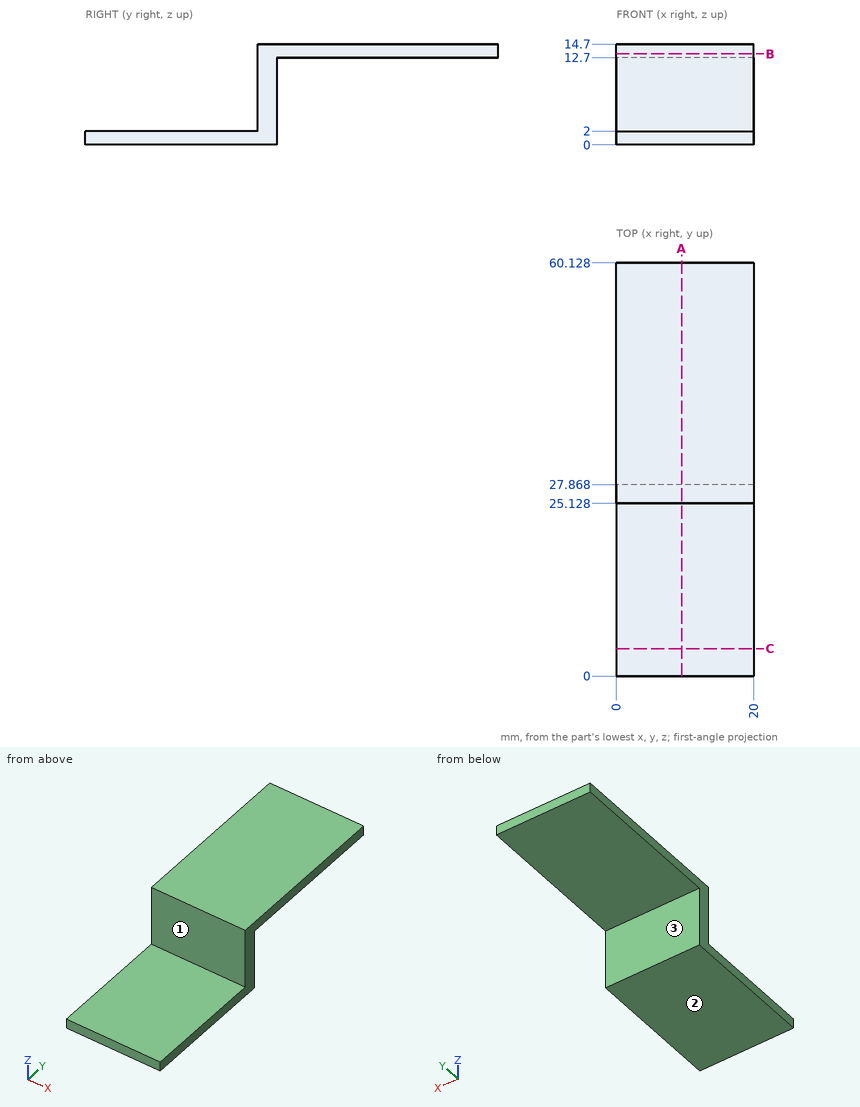
Could you check a few things on this drawing? It's one solid part, dimensions in mm from its lowest x, y, z. A direction names the side the tool comes from. Give positions to 0.01 mm unless a question says otherwise; leave off trailing zeros. Write each loop counter-clockwise with the first axis right and the second up, starting at its lowest first coordinate (ties: lowest second). Pieces come first, ordered by that corner, then holes. Notation, with made-up numbers: M 36,-2.5 L 95,-2.5 A19 cw 95,30.5 Z; hole C -17,57 d1. An arc over 180 degrees is marked long. Put each result on its own line as item: value. Start each with the question number.
Item 1: Will these pins go through, and if not, where does the flat tip stop? pin 1 (10 mm diameter, centred on x = 12, y = 15, fed in from +Z); pin 2 (2 mm diameter, centred on x = 17, z = 4, fed in from -Y); pin 3 (2 mm diameter, centred on x = 3, y = 25, fed in from -Z); pin 4 (6.5 mm diameter, centred on x = 10, z = 7.5, fed in from +Y).
Item 2: On a 3-axis mill with a long thin cutter (end or side, diameter ignored), from which of +Z, -Z, +X, -X, +Y, -Y can I reach the whole of each face in a straight line? I mean the marked faces 1, 2 and 3. Say none if no direction works.
Item 3: If we section it at C-C, the plane y = 4: Write out the boundary of the cut face in (x, z).
Item 4: I need wall thicknesses on L1, parallel to Z at x = 10.25, y = 32.5; L2, parallel to Y at x = 13.75, z = 9; L3, parallel to Y at x = 8.5, z = 0.75. Which ranges of each line are inside material? Lowest first, please. Write a range as from..to.
Item 5: If we section it at A-A, the plane x = 9.5: Write out the boundary of the cut face in (y, z).
Item 6: If we section it at B-B, the plane z = 13.25: Write out the boundary of the cut face in (x, y).
Values:
1. pin 1: z = 2
1. pin 2: y = 25.13
1. pin 3: z = 0
1. pin 4: y = 27.87
2. face 1: +Z, +X, -X, -Y
2. face 2: -Z, +X, -X, +Y, -Y
2. face 3: -Z, +X, -X, +Y
3. outline: M 0,0 L 20,0 L 20,2 L 0,2 Z
4. L1: 12.7..14.7
4. L2: 25.13..27.87
4. L3: 0..27.87
5. outline: M 0,0 L 27.87,0 L 27.87,12.7 L 60.13,12.7 L 60.13,14.7 L 25.13,14.7 L 25.13,2 L 0,2 Z
6. outline: M 0,25.13 L 20,25.13 L 20,60.13 L 0,60.13 Z
